Autodesk Inventor part; units mm, degrees
ref_plane "YZ Plane" through (0, 0, 0) normal (1, 0, 0) x (0, 1, 0)
ref_plane "XZ Plane" through (0, 0, 0) normal (0, 1, 0) x (-1, 0, 0)
ref_plane "XY Plane" through (0, 0, 0) normal (0, 0, 1) x (1, 0, 0)
sketch "Sketch1" plane through (0, 0, 0) normal (0, 0, 1) x (1, 0, 0)
  line L0 (0, 0) -> (0, 17.5) construction
  line L1 (0, 0) -> (-10, 0)
  line L2 (0, 0) -> (10, 0)
  line L3 (-10, 0) -> (-10, 4.6)
  line L4 (-10, 4.6) -> (-6.1, 8.5)
  line L5 (-6.1, 8.5) -> (-6.1, 9)
  line L6 (-6.1, 9) -> (-10, 12.9)
  line L7 (-10, 12.9) -> (-10, 15.4)
  line L8 (-10, 15.4) -> (-7.9, 17.5)
  line L9 (-7.9, 17.5) -> (0, 17.5)
  line L10 (10, 0) -> (10, 4.6)
  line L11 (10, 4.6) -> (6.1, 8.5)
  line L12 (6.1, 8.5) -> (6.1, 9)
  line L13 (6.1, 9) -> (10, 12.9)
  line L14 (10, 12.9) -> (10, 15.4)
  line L15 (10, 15.4) -> (7.9, 17.5)
  line L16 (7.9, 17.5) -> (0, 17.5)
  dimension "d0" = 17.5
  dimension "d1" = 20
  dimension "d2" = 4.6
  dimension "d3" = 8.5
  dimension "d8" = 135
  dimension "d9" = 0.5
  dimension "d10" = 135
  dimension "d11" = 2.5
extrude "Extrusion1" add sketch "Sketch1" along normal blind 300
sketch "Sketch2" plane through (0, 0, 0) normal (0, 1, 0) x (-1, 0, 0)
  line L0 (0, 0) -> (0, 20) construction
  line L1 (0, 20) -> (0, 80) construction
  circle A0 centre (0, 20) radius 4.75
  circle A1 centre (0, 20) radius 3
  dimension "d14" = 20
  dimension "d15" = 60
  dimension "d16" = 9.5
  dimension "d17" = 6
extrude "Extrusion2" cut sketch "Sketch2" along normal through all contours A1
extrude "Extrusion3" cut sketch "Sketch2" against normal blind 8.5 from surface at 17.5
pattern_linear "Rectangular Pattern1" count 9 spacing 60 along (0, 0, 1) of "Extrusion2", "Extrusion3"
properties part number "HGR20 500mm"
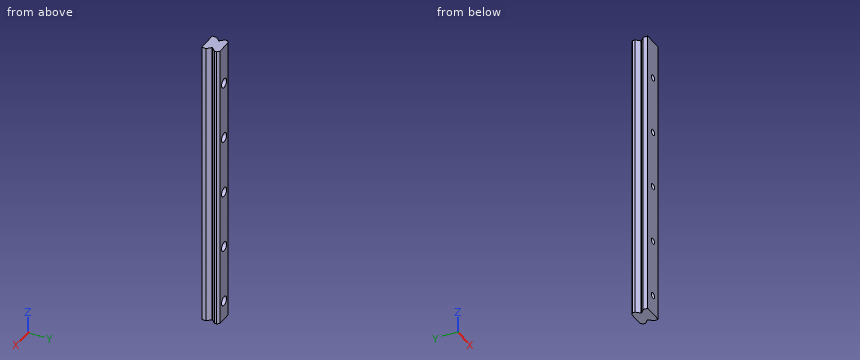
Could you check a few things on this model? Use its own coordinates, in mm. Give positions to 0.01 mm unless a question says otherwise; leave off trailing zeros. Order: outer loops, then holes, each group sorted by start corner. A loop starts at its lowest first (then second) coordinate and runs counter-clockwise, first axis right, second up.
1. Suppose I cut it at C-C (x = -0.25). Give the number of separate pieces and of enclosed holes in the cut face, plus the area to 3 significant figures.
2. Suppose I cut it at B-B (z = 152.5). List the corners of the cut face in (x, y) for me, plus the area to 3 significant figures.
3. Will these pins go through, and if not, where does the flat tip stop? P1, Ø5, axis at x = 0, z = 200, coming from the +Y side; P2, Ø8.5, axis at x = 0, z = 260, coming from the +Y side; P3, Ø0.6, axis at y = 8.5, z = 205, coming from the -X side.
4. Suppose I cut it at A-A (z = 200). List the corners of the cut face in (x, y) for me.
5. I need wall thicknesses on L1, parallel to Z at x = 0, y = 11; L2, parallel to Z at x = 3, y = 16.75; L3, parallel to X at y = 4, z = 260. Which ranges of each line are inside material? Lowest first, please.
Solved:
1. separate pieces: 6
1. enclosed holes: 0
1. area: 4,580 mm2
2. outline: (-10, 0) - (10, 0) - (10, 4.6) - (6.1, 8.5) - (6.1, 9) - (10, 12.9) - (10, 15.4) - (7.9, 17.5) - (-7.9, 17.5) - (-10, 15.4) - (-10, 12.9) - (-6.1, 9) - (-6.1, 8.5) - (-10, 4.6) - close
2. area: 311 mm2
3. P1: passes through
3. P2: stops at y = 9
3. P3: stops at x = -6.4
4. outline: (-10, 0) - (-3, 0) - (-3, 9) - (-4.75, 9) - (-4.75, 17.5) - (-7.9, 17.5) - (-10, 15.4) - (-10, 12.9) - (-6.1, 9) - (-6.1, 8.5) - (-10, 4.6) - close; (3, 0) - (10, 0) - (10, 4.6) - (6.1, 8.5) - (6.1, 9) - (10, 12.9) - (10, 15.4) - (7.9, 17.5) - (4.75, 17.5) - (4.75, 9) - (3, 9) - close
5. L1: z = 0 to 15.25, 24.75 to 75.25, 84.75 to 135.25, 144.75 to 195.25, 204.75 to 255.25, 264.75 to 300
5. L2: z = 0 to 16.32, 23.68 to 76.32, 83.68 to 136.32, 143.68 to 196.32, 203.68 to 256.32, 263.68 to 300
5. L3: x = -10 to -3, 3 to 10
